Can you work these out from the drawing? Everything is in mm from the part's minimum corner. A direction names the side the tool comes from. Round coordinates to 2 decimals unless told otherwise and drop trailing zeros. Write each loop counter-clockwise with the first axis right and the second up, starting at its lowest first coordinate (ties: lowest second). Pieces come first, ordered by that corner, then holes. Notation, with made-up numbers: (9.5, 60) - (55.5, 60) arc R19 ccw to (55.5, 67) - close; hole circle Ø5 at (-14.75, 82.5). An arc over 180 degrees is marked (long way). One line per item, written item: value. Start each with the question number.
Item 1: For P1, Ø1.5, axis at y = 16, z = 105, coming from the -X side, with a flat end and sliding along its axis, tell me the tip position at first contact or that it passes through.
Item 2: Imagine slicing it at D-D, the plane z = 89. Please give me the cut outline in (x, y) (1 decimal), then the cut area to 3 significant figures.
Item 3: Thinking about a two-plate mould opening in X: for the marked faces 1, 2 and 3, which applies, released by +X, released by -X, zero draft, split by the parting line, or undercut?
Item 4: If I drill on line 1 (X direction, y = 23.75, z = 68.5); line 2 (Z direction, x = 82.5, y = 7) (1 decimal); line 3 (X direction, y = 4.5, z = 104.5), over which ranges is the centre line in solid material (lowest first)?
Item 5: Imagine slicing it at C-C, the plane x = 54.5. Please give me the cut outline in (y, z).
Item 6: For the marked faces 4 and 5, which set-ups out of +Z, -Z, +X, -X, +Y, -Y let a thin tool reach every point of the face, with its end or its side?
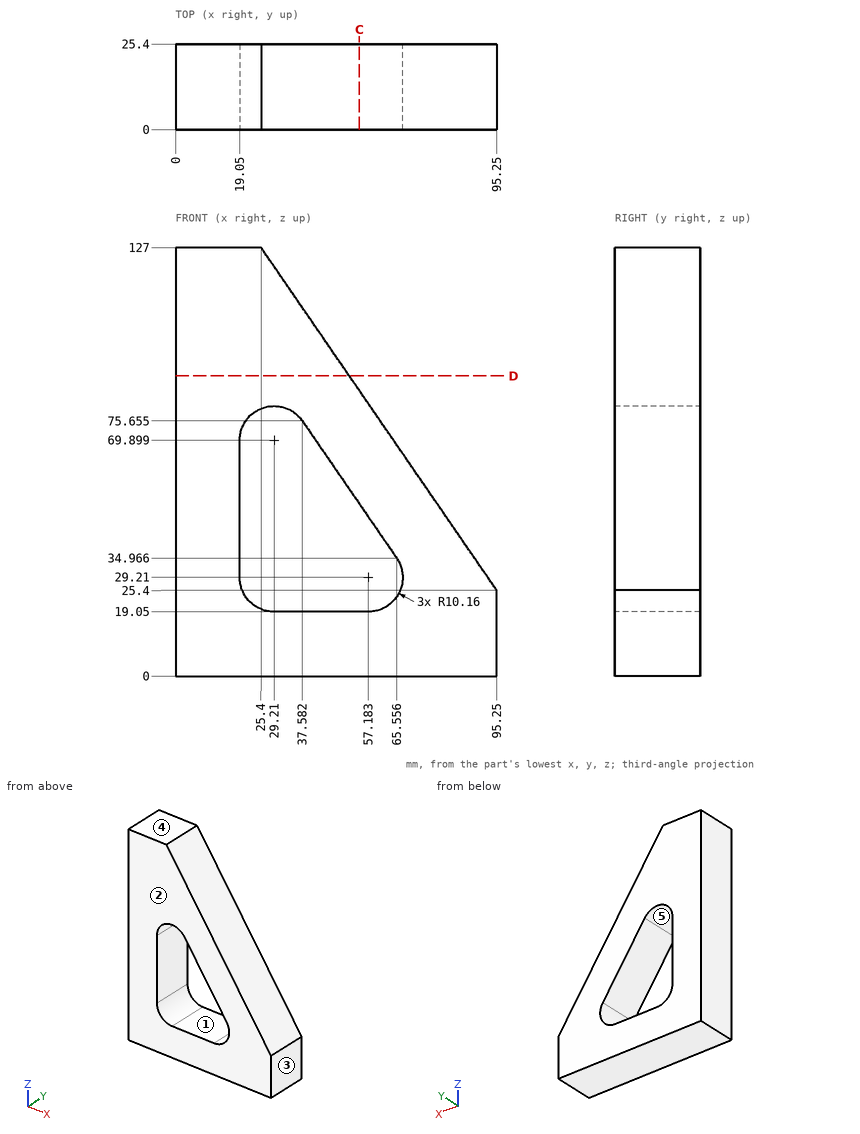
Values follow:
1. P1: stops at x = 0
2. outline: (0, 0) - (51.5, 0) - (51.5, 25.4) - (0, 25.4) - close
2. area: 1,310 mm^2
3. face 1: undercut
3. face 2: zero draft
3. face 3: released by +X
4. line 1: x = 0 to 19.05, 42.5 to 65.62
4. line 2: z = 0 to 43.9
4. line 3: x = 0 to 40.87
5. outline: (0, 0) - (25.4, 0) - (25.4, 19.05) - (0, 19.05) - close; (0, 51.05) - (25.4, 51.05) - (25.4, 84.67) - (0, 84.67) - close
6. face 4: +Z, +X, -X, +Y, -Y
6. face 5: +Y, -Y
